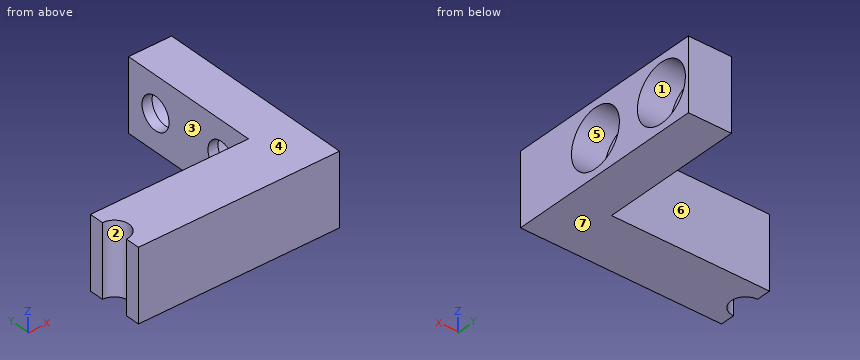
Autodesk Inventor part; units mm, degrees
ref_plane "YZ Plane" through (0, 0, 0) normal (1, 0, 0) x (0, 1, 0)
ref_plane "XZ Plane" through (0, 0, 0) normal (0, 1, 0) x (-1, 0, 0)
ref_plane "XY Plane" through (0, 0, 0) normal (0, 0, 1) x (1, 0, 0)
sketch "Sketch1" plane through (0, 0, 0) normal (0, 0, 1) x (1, 0, 0)
  line L0 (0, 20) -> (6, 20)
  line L1 (6, 20) -> (6, 0)
  line L2 (6, 0) -> (0, 0)
  line L3 (0, 0) -> (0, 20)
  line L4 (6, 0) -> (-22, 0)
  line L5 (-22, 0) -> (-22, -8)
  line L6 (-22, -8) -> (6, -8)
  line L7 (6, -8) -> (6, 0)
  circle A0 centre (-22, -4) radius 2
  point P0 (0, 0)
  point P1 (-22, -2)
  point P2 (-22, -6)
  dimension "d0" = 20
  dimension "d1" = 6
  dimension "d2" = 4
  dimension "d3" = 8
  dimension "d4" = 22
extrude "Extrusion1" add sketch "Sketch1" along normal blind 10 contours L0 L1 L2 L3 | L2 L7 L6 L5 A0 L4
sketch "Sketch2" plane through (6, -8, 0) normal (1, 0, 0) x (0, 0, -1)
  line L0 (0, 28) -> (-10, 28)
  point P0 (0, 8)
  point P1 (-5, 12.5)
  point P2 (-5, 23.5)
  point P3 (-5, 28)
  dimension "d14" = 11
  dimension "d15" = 4.5
hole "Hole1" at (6, 15.5, 5) at (6, 4.5, 5) direction (-1, 0, 0) diameter 4.5 end through all counterbore diameter 8 counterbore depth 4.6
properties part number "Gripper arm" material "Steel"
Can you work these out from the model? Positions are in its coordinate system, mm. Face numbers are marked on the shaded views. A direction names the side the tool comes from. Round coordinates to 2 decimals unless told otherwise and drop trailing zeros. Loops run counter-clockwise (first coordinate to the right, second up) from the corner with the lowest first, then second, coordinate; pieces in that order, holes last.
Item 1: If we mould it in two halves opening along Z, with no side actions, what happens to the marked faces 4, 5, 6 and 7? For each: +Z half, -Z half, draft (parallel to the pull), parting line (faces both ways), or undercut.
Item 2: Which directions (+Z, -Z, +X, -X, +Y, -Y) give clear straight access to the entire face, cutting with the end or side of a thin tool? Please do the marked faces 1, 2 and 3.
Item 3: Suppose I cut it at D-D, the plane x = -7.75. Write out the boundary of the cut face in (y, z).
Item 4: Please list where these lines run through material, in increasing order: L1, parallel to Y at x = 1.05, z = 5; L2, parallel to Z at x = 0.45, y = 15.5; L3, parallel to Z at x = 4.2, y = 15.5.
Item 5: Will these pins go through, and if not, where does the flat tip stop? pin 1 Ø4 at (y, z) = (5, 5) entering from +X; pin 2 Ø4 at (x, z) = (-5, 4) entering from +Y.
Item 6: Suppose I cut it at C-C, the plane y = -4. Write out the boundary of the cut face in (x, z), then the cut area to 3 significant figures.
Item 7: Suppose I cut it at A-A, the plane z = 5. Write out the boundary of the cut face in (x, y), then the cut area to 3 significant figures.
Item 8: Suppose I cut it at B-B, the plane y = 15.5. Write out the boundary of the cut face in (x, z).
Reported:
1. face 4: +Z half
1. face 5: undercut
1. face 6: draft
1. face 7: -Z half
2. face 1: +X
2. face 2: +Z, -Z, -X
2. face 3: +Z, -Z, -X, +Y
3. outline: (-8, 0) - (0, 0) - (0, 10) - (-8, 10) - close
4. L1: y = -8 to 2.25, 6.75 to 13.25, 17.75 to 20
4. L2: z = 0 to 2.75, 7.25 to 10
4. L3: z = 0 to 1, 9 to 10
5. pin 1: stops at x = 1.4
5. pin 2: stops at y = 0
6. outline: (-20, 0) - (6, 0) - (6, 10) - (-20, 10) - close
6. area: 260 mm2
7. outline: (-22, -8) - (6, -8) - (6, 0.5) - (1.4, 0.5) - (1.4, 2.25) - (0, 2.25) - (0, 0) - (-22, 0) - (-22, -2) arc R2 cw to (-22, -6) - close; (0, 6.75) - (1.4, 6.75) - (1.4, 8.5) - (6, 8.5) - (6, 11.5) - (1.4, 11.5) - (1.4, 13.25) - (0, 13.25) - close; (0, 17.75) - (1.4, 17.75) - (1.4, 19.5) - (6, 19.5) - (6, 20) - (0, 20) - close
7. area: 252 mm2
8. outline: (0, 0) - (6, 0) - (6, 1) - (1.4, 1) - (1.4, 2.75) - (0, 2.75) - close; (0, 7.25) - (1.4, 7.25) - (1.4, 9) - (6, 9) - (6, 10) - (0, 10) - close
